Can you work these out from the model? Positions are in its coordinate system, mm. A direction names the side the tool comes from. Coordinates: 2 decimals unless noted, no trailing zeros. Order: outer loops, then holes, each group sorted by start corner. A loop starts at its lowest first (then second) coordinate and runs counter-clockwise, first axis right, second up. Notation, with made-up numbers: (79.5, -33) -> (124.5, -33) arc R27 cw to (124.5, -2) -> close; hole circle Ø2 at (81, 3). An arc over 180 degrees is marked (long way). Use a Markdown table: item, result. Add a question column.
1. Suppose I cut it at C-C, the plane x = 72.5. List the corners of the cut face in (y, z) for me.
2. We'd pull the mould along Z, two halves only. Please class faces 1 (the flat face through (-1, 7, -35)), 2 (the flat face through (75, 7, 0)), 3 (the flat face through (2, 15, -16)): pulls with the +Z half, pulls with the -Z half, needs draft (parallel to the pull), parting line crosses it, or undercut.
3. Suppose I cut it at A-A, the plane y = 10.5. List the corners of the cut face in (x, z) for me, then the cut area to 3 significant figures.
4. If I drill on line 1 along Z through (x, y) = (-11.5, 4.75); line 2 along X through (y, z) = (5.5, -0.5); line 3 along X through (y, z) = (14, 3), over which ranges is the centre line in solid material (lowest first)? Write a range as from..to.
5. Suppose I cut it at B-B, the plane z = 0. List the corners of the cut face in (x, y) for me.
6. For faces 4 (the flat face through (-1, 7, -15)), 5 (the flat face through (1, 7, 35)), which set-ups out of +Z, -Z, +X, -X, +Y, -Y let a thin tool reach every point of the face, with its end or its side?
7. For pin 1 Ø2 at (y, z) = (8, -12) entering from +X; pin 2 Ø1.5 at (x, z) = (-13, -13) entering from +Y; pin 3 Ø7.5 at (y, z) = (11, -5.5) entering from -X; pin 4 Ø1.5 at (y, z) = (13, 14.5) entering from -X, each with a flat end and sliding along its axis, tell me the tip position at first contact or that it passes through.
```python
from build123d import *

# Parameters (mm, degrees)
SKETCH1_W           = 150
SKETCH1_H           = 30
BOSS_EXTRUDE1_DEPTH = 15


with BuildPart() as part:
    # Sketch1 → Boss-Extrude1 (new body)
    with BuildSketch(Plane(origin=(0, 0, 0), x_dir=(1, 0, 0), z_dir=(0, 1, 0))):
        with BuildLine():
            Line((-75, 35), (75, 35))
            ThreePointArc((75, 35), (110, 0), (75, -35))
            Line((75, -35), (-75, -35))
            ThreePointArc((-75, -35), (-110, 0), (-75, 35))
        make_face()
        Rectangle(SKETCH1_W, SKETCH1_H, mode=Mode.SUBTRACT)
    extrude(amount=BOSS_EXTRUDE1_DEPTH)


solid = part.part
```
Worked out:
| question | item | result |
|---|---|---|
| 1 | outline | (0, -35) -> (15, -35) -> (15, -15) -> (0, -15) -> close; (0, 15) -> (15, 15) -> (15, 35) -> (0, 35) -> close |
| 2 | face 1 | pulls with the -Z half |
| 2 | face 2 | undercut |
| 2 | face 3 | needs draft |
| 3 | outline | (-75, -35) -> (75, -35) arc R35 ccw to (75, 35) -> (-75, 35) arc R35 ccw to start; hole (-75, -15) -> (75, -15) -> (75, 15) -> (-75, 15) -> close |
| 3 | area | 9,850 mm² |
| 4 | line 1 | z = -35..-15, 15..35 |
| 4 | line 2 | x = -110..-75, 75..110 |
| 4 | line 3 | x = -109.87..-75, 75..109.87 |
| 5 | outline | (-110, 0) -> (-75, 0) -> (-75, 15) -> (-110, 15) -> close; (75, 0) -> (110, 0) -> (110, 15) -> (75, 15) -> close |
| 6 | face 4 | +Y, -Y |
| 6 | face 5 | +Z, +X, -X, +Y, -Y |
| 7 | pin 1 | stops at x = 108.23 |
| 7 | pin 2 | passes through |
| 7 | pin 3 | stops at x = -109.96 |
| 7 | pin 4 | stops at x = -107.19 |
